```python
from build123d import *

# Parameters (mm, degrees)
SKETCH2_W           = 110
SKETCH2_H           = 8
BOSS_EXTRUDE1_DEPTH = 12
LPATTERN1_COUNT     = 5
LPATTERN1_PITCH     = 22
SKETCH4_R           = 2
BOSS_EXTRUDE2_DEPTH = 4
BOSS_EXTRUDE2_TAPER = 1


with BuildPart() as part:
    # Sketch2 → Boss-Extrude1 (new body)
    with BuildSketch(Plane.XY):
        with Locations((55, 4)):
            Rectangle(SKETCH2_W, SKETCH2_H)
    extrude(amount=-BOSS_EXTRUDE1_DEPTH)

    # Sketch3 → Cut-Revolve1 (revolve, cut)
    with BuildSketch(Plane.XY):
        Polygon((8, 3), (8.9, 3), (8.9, 5), (2, 5), (2, 6), (11, 6), (11, 0), (8.9, 0), align=None)
    cut_revolve1 = revolve(axis=Axis((11, 6, 0), (0, -1, 0)), mode=Mode.SUBTRACT)

    # LPattern1: Cut-Revolve1 ×5
    with Locations(*[(i * LPATTERN1_PITCH, 0, 0) for i in range(1, LPATTERN1_COUNT)]):
        add(cut_revolve1, mode=Mode.SUBTRACT)

    # Sketch4 → Boss-Extrude2 (add)
    with BuildSketch(Plane.XY):
        with Locations((22, 3)):
            Circle(SKETCH4_R)
        with Locations((88, 3)):
            Circle(SKETCH4_R)
    extrude(amount=BOSS_EXTRUDE2_DEPTH, taper=BOSS_EXTRUDE2_TAPER)


solid = part.part
```
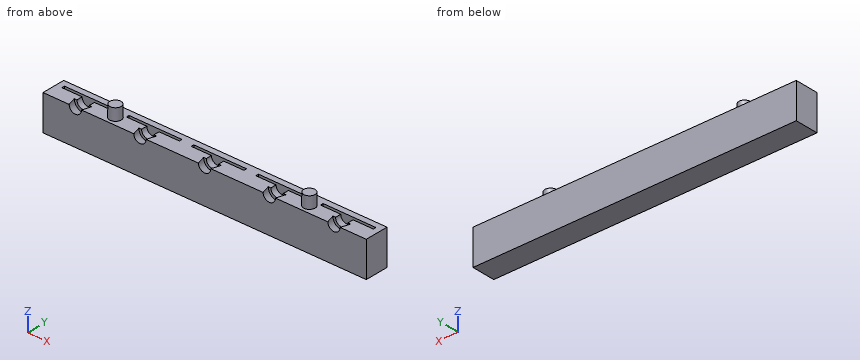
The model under review builds one solid part; all positions refer to its coordinate system, in mm. Coordinates: 2 decimals unless noted, no trailing zeros. Write each loop counter-clockwise with the first axis right and the second up, starting at its lowest first coordinate (ties: lowest second). Pieces come first, ordered by that corner, then holes. Notation, with made-up numbers: (29, 56) -> (34, 56) arc R26 cw to (34, 70) -> close; hole circle Ø2 at (20, -1.5). An arc over 180 degrees is marked (long way). One line per item, written item: value. Start each with the question number.
Q1. Clearance check with a flat-ended pin moving along its axis: P1, Ø2.5, axis at x = 36.5, y = 6, coming from the +Z side. State where the tip first meets the part, or that it passes through.
Q2. Add section D-D, the plane x = 69. Give the boundary of the cut face in (y, z).
Q3. Add section C-C, the plane z = 1.25. Give the boundary of the cut face in (x, y).
Q4. Add section B-B, the plane z = -7. Give the boundary of the cut face in (x, y), then the cut area to 3 significant figures.
Q5. To check wall thickness, follow probe 1 along X at (y, z) = (4.5, -0.25); probe 2 along Y at (x, z) = (25.5, -1.75); probe 3 along Z at (x, y) = (102.5, 6.75). State the ranges of each line that lie inside material, in increasing order.
Q6. Add section A-A, the plane x = 55. Give the boundary of the cut face in (y, z).
Response:
1. P1: z = 0
2. outline: (0, -12) -> (8, -12) -> (8, 0) -> (6, 0) -> (6, -4.12) -> (5, -4.12) -> (5, 0) -> (0, 0) -> close
3. outline: circle Ø3.96 at (22, 3); circle Ø3.96 at (88, 3)
4. outline: (0, 0) -> (110, 0) -> (110, 8) -> (0, 8) -> close; hole (5.34, 5) -> (16.66, 5) -> (16.66, 6) -> (5.34, 6) -> close; hole (27.34, 5) -> (38.66, 5) -> (38.66, 6) -> (27.34, 6) -> close; hole (49.34, 5) -> (60.66, 5) -> (60.66, 6) -> (49.34, 6) -> close; hole (71.34, 5) -> (82.66, 5) -> (82.66, 6) -> (71.34, 6) -> close; hole (93.34, 5) -> (104.66, 5) -> (104.66, 6) -> (93.34, 6) -> close
4. area: 823 mm²
5. probe 1: 0 to 8.91, 13.09 to 30.91, 35.09 to 52.91, 57.09 to 74.91, 79.09 to 96.91, 101.09 to 110
5. probe 2: 0 to 5, 6 to 8
5. probe 3: -12 to 0
6. outline: (0, -12) -> (8, -12) -> (8, 0) -> (6, 0) -> (6, -9) -> (5, -9) -> (5, -2.1) -> (3, -2.1) -> (3, -3) -> (0, -2.1) -> close
